Read the model definition and answer for the solid it produces. Units are mm, in the model's axes. Face numbers are marked on the shaded views. A direction names the side the tool comes from. Coordinates: 2 decimals unless noted, no trailing zeros. Write each loop counter-clockwise with the first axis right and the second up, starting at its lowest first coordinate (ties: lowest second). Pieces come first, ordered by that corner, then holes. Notation, with made-up numbers: (63, 22.25) -> (84, 22.25) arc R24 ccw to (84, 58.25) -> close; hole circle Ø6 at (43.25, 17.5). An arc over 180 degrees is marked (long way). Write item = value, one per line. Start each with the question number.
1) A tool of negligible diameter and unlimited length cuts with its end or side. For the marked faces 1 and 2, from which of +Z, -Z, +X, -X, +Y, -Y can it reach the whole face along a straight path? Write none if from no direction.
2) Find the intervals of material crossed by line 1 along Y through (x, z) = (0, 3) (3 decimals); line 2 along X through (y, z) = (5.5, 9.5); line 3 along X through (y, z) = (-8.5, 17.5), in increasing order. Write a range as from..to.
3) Section A-A (z = 7) is taken. Determine the outline of the cut face in (x, y) (3 decimals), plus the area to 3 significant figures.
4) For a pull along Y with two mould halves and no side action, classify the marked faces 3, 4 and 5 as released by +Y, released by -Y, zero draft, split by the parting line, or undercut.
5) Flat-ended cylindrical pins translate along their axes: pin 1 Ø1.5 at (x, y) = (12.99, 7.5) entering from -Z; pin 2 Ø10 at (x, y) = (6, -11.5) entering from +Z; pin 3 Ø8 at (y, z) = (20, 10) entering from +X; pin 4 Ø5 at (x, z) = (-38, 13.5) entering from -Y. Find the tip coordinate at first contact, or state that the pin passes through.
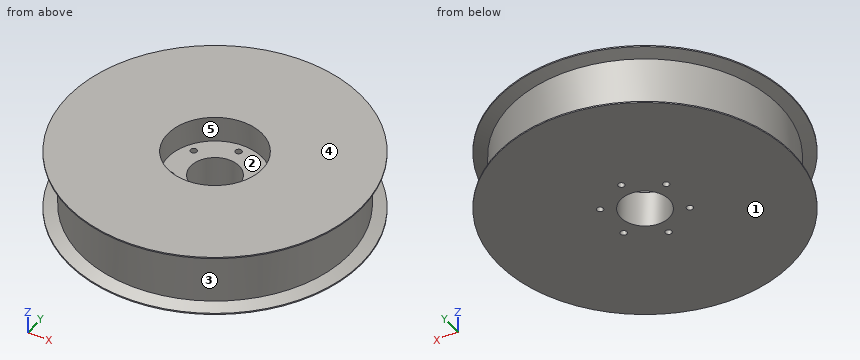
from build123d import *

# Parameters (mm, degrees)
SKETCH_1_R          = 57.5
SKETCH_1_R_2        = 9.5
EXTRUDE_1_DEPTH     = 24.2
SKETCH_3_R          = 18.5
SKETCH_3_R_2        = 9.5
CUT_EXTRUDE_2_DEPTH = 10
SKETCH_4_R          = 1.25
CUT_EXTRUDE_3_DEPTH = 25.2


with BuildPart() as part:
    # 草圖1 → 填料-伸長1 (new body)
    with BuildSketch(Plane.XY):
        Circle(SKETCH_1_R)
        Circle(SKETCH_1_R_2, mode=Mode.SUBTRACT)
    extrude(amount=EXTRUDE_1_DEPTH)

    # 草圖3 → 除料-伸長2 (cut)
    with BuildSketch(Plane.XY.offset(24.2)):
        Circle(SKETCH_3_R)
        Circle(SKETCH_3_R_2, mode=Mode.SUBTRACT)
    extrude(amount=-CUT_EXTRUDE_2_DEPTH, mode=Mode.SUBTRACT)

    # 草圖4 → 除料-伸長3 (cut, through all)
    with BuildSketch(Plane(origin=(0, 0, 0), x_dir=(-1, 0, 0), z_dir=(0, 0, -1))):
        with Locations((0, 15)):
            Circle(SKETCH_4_R)
        with Locations((12.990381057, -7.5)):
            Circle(SKETCH_4_R)
        with Locations((-12.990381057, -7.5)):
            Circle(SKETCH_4_R)
        with Locations((12.990381057, 7.5)):
            Circle(SKETCH_4_R)
        with Locations((0, -15)):
            Circle(SKETCH_4_R)
        with Locations((-12.990381057, 7.5)):
            Circle(SKETCH_4_R)
    extrude(amount=-CUT_EXTRUDE_3_DEPTH, mode=Mode.SUBTRACT)

    # 草圖5 → 除料-旋轉1 (revolve, cut)
    with BuildSketch(Plane(origin=(0, 0, 0), x_dir=(1, 0, 0), z_dir=(0, 1, 0))):
        Polygon((57.5, -23.7), (52.555, -22.35), (52.555, -1.85), (57.5, -0.5), align=None)
    revolve(axis=Axis((0, 0, 0), (0, 0, 1)), mode=Mode.SUBTRACT)


solid = part.part
Answer key:
q1.face_1 = -Z, +X, -X, +Y, -Y
q1.face_2 = +Z
q2.line_1 = -52.555..-16.25, -13.75..-9.5, 9.5..13.75, 16.25..52.555
q2.line_2 = -52.27..-7.75, 7.75..52.27
q2.line_3 = -51.86..-16.43, 16.43..51.86
q3.outline = circle Ø105.11 at (0, 0); hole circle Ø2.5 at (-12.99, -7.5); hole circle Ø2.5 at (-12.99, 7.5); hole circle Ø19 at (0, 0); hole circle Ø2.5 at (0, -15); hole circle Ø2.5 at (0, 15); hole circle Ø2.5 at (12.99, -7.5); hole circle Ø2.5 at (12.99, 7.5)
q3.area = 8,360 mm^2
q4.face_3 = split by the parting line
q4.face_4 = zero draft
q4.face_5 = undercut
q5.pin_1 = through
q5.pin_2 = 14.2
q5.pin_3 = 50.06
q5.pin_4 = -38.75
